Geometry check sheet. Reference: the model listing, model coordinates, mm. A direction names the side the tool comes from. Give positions to 0.01 mm unless a question says otherwise; leave off trailing zeros. Write each loop counter-clockwise with the first axis right and the second up, starting at its lowest first coordinate (ties: lowest second). Pieces come first, ordered by that corner, then holes. Notation, with made-up numbers: (82, 68.25) -> (114, 68.25) arc R20 cw to (114, 93.25) -> close; hole circle Ø5 at (38.25, 13). An arc over 180 degrees is marked (long way). One line per item, written item: value.
from build123d import *

# Parameters (mm, degrees)
F0_W      = 76.2
F0_H      = 38.1
F1_DEPTH  = 19.05
F3_DEPTH  = 3.048
F4_R      = 8.255
F5_DEPTH  = 4.572
F6_R      = 2.159
F7_DEPTH  = 12.7
F8_R      = 5.08
F9_DEPTH  = 12.7
F11_DEPTH = 3.048


with BuildPart() as f1:
    # F0 (on Top) → F1 (new body)
    with BuildSketch(Plane.XY):
        with Locations((38.1, 19.05)):
            Rectangle(F0_W, F0_H)
    extrude(amount=F1_DEPTH)

    # F2 (on face) → F3 (cut)
    with BuildSketch(Plane.XY.offset(19.05)):
        with BuildLine():
            ThreePointArc((7.0865621097, 27.8874175237), (11.4470908204, 28.4614920193), (13.4779330423, 32.3627036302))
            ThreePointArc((13.4779330423, 32.3627036302), (12.6166446532, 35.0943614084), (10.3443039749, 36.8379897367))
            ThreePointArc((10.3443039749, 36.8379897367), (4.2401469358, 33.9915745628), (7.0865621097, 27.8874175237))
        make_face()
        with BuildLine():
            ThreePointArc((10.3443039749, 36.8379897367), (12.6166446532, 35.0943614084), (13.4779330423, 32.3627036302))
            ThreePointArc((13.4779330423, 32.3627036302), (11.4470908204, 28.4614920193), (7.0865621097, 27.8874175237))
            Line((7.0865621097, 27.8874175237), (35.7283931912, 17.4626435552))
            ThreePointArc((35.7283931912, 17.4626435552), (32.5947641238, 21.9379296617), (35.7283931912, 26.4132157682))
            Line((35.7283931912, 26.4132157682), (37.3572641238, 27.0060763031))
            Line((37.3572641238, 27.0060763031), (10.3443039749, 36.8379897367))
        make_face()
        with BuildLine():
            Line((64.3702242728, 36.8379897367), (37.3572641238, 27.0060763031))
            Line((37.3572641238, 27.0060763031), (38.9861350564, 26.4132157682))
            ThreePointArc((38.9861350564, 26.4132157682), (41.2584757347, 24.6695874398), (42.1197641238, 21.9379296617))
            ThreePointArc((42.1197641238, 21.9379296617), (41.2584757347, 19.2062718836), (38.9861350564, 17.4626435552))
            Line((38.9861350564, 17.4626435552), (67.627966138, 27.8874175237))
            ThreePointArc((67.627966138, 27.8874175237), (61.5238090989, 30.7338326977), (64.3702242728, 36.8379897367))
        make_face()
        with BuildLine():
            Line((38.9861350564, 26.4132157682), (37.3572641238, 27.0060763031))
            Line((37.3572641238, 27.0060763031), (35.7283931912, 26.4132157682))
            ThreePointArc((35.7283931912, 26.4132157682), (37.3572641238, 26.7004296617), (38.9861350564, 26.4132157682))
        make_face()
        with BuildLine():
            ThreePointArc((35.7283931912, 26.4132157682), (32.5947641238, 21.9379296617), (35.7283931912, 17.4626435552))
            ThreePointArc((35.7283931912, 17.4626435552), (37.3572641238, 17.1754296617), (38.9861350564, 17.4626435552))
            ThreePointArc((38.9861350564, 17.4626435552), (41.2584757347, 19.2062718836), (42.1197641238, 21.9379296617))
            ThreePointArc((42.1197641238, 21.9379296617), (41.2584757347, 24.6695874398), (38.9861350564, 26.4132157682))
            ThreePointArc((38.9861350564, 26.4132157682), (37.3572641238, 26.7004296617), (35.7283931912, 26.4132157682))
        make_face()
        with BuildLine():
            ThreePointArc((70.7615952054, 32.3627036302), (68.7307529835, 36.2639152412), (64.3702242728, 36.8379897367))
            ThreePointArc((64.3702242728, 36.8379897367), (61.5238090989, 30.7338326977), (67.627966138, 27.8874175237))
            ThreePointArc((67.627966138, 27.8874175237), (69.9003068163, 29.6310458521), (70.7615952054, 32.3627036302))
        make_face()
    extrude(amount=-F3_DEPTH, mode=Mode.SUBTRACT)

    # F4 (on face) → F5 (cut)
    with BuildSketch(Plane.XY.offset(19.05)):
        with Locations((56.4142079383, 17.0484144696)):
            Circle(F4_R)
    extrude(amount=-F5_DEPTH, mode=Mode.SUBTRACT)

    # F6 (on face) → F7 (cut)
    with BuildSketch(Plane.XY.offset(14.478)):
        with Locations((56.4142079383, 17.0484144696)):
            Circle(F6_R)
    extrude(amount=-F7_DEPTH, mode=Mode.SUBTRACT)

    # F8 (on face) → F9 (cut)
    with BuildSketch(Plane.XY.offset(16.002)):
        with Locations((37.3572641238, 21.9379296617)):
            Circle(F8_R)
    extrude(amount=-F9_DEPTH, mode=Mode.SUBTRACT)

    # F10 (on face) → F11 (cut)
    with BuildSketch(Plane.XY.offset(19.05)):
        with BuildLine():
            ThreePointArc((7.0865621097, 27.8874175237), (4.8142214313, 29.6310458521), (3.9529330423, 32.3627036302))
            Line((3.9529330423, 32.3627036302), (3.9529330423, 0))
            Line((3.9529330423, 0), (70.7615952054, 0))
            Line((70.7615952054, 0), (70.7615952054, 32.3627036302))
            ThreePointArc((70.7615952054, 32.3627036302), (69.9003068163, 29.6310458521), (67.627966138, 27.8874175237))
            Line((67.627966138, 27.8874175237), (59.1989824769, 24.819518366))
            Line((59.1989824769, 24.819518366), (49.2857775794, 21.2114068571))
            Line((49.2857775794, 21.2114068571), (38.9861350564, 17.4626435552))
            ThreePointArc((38.9861350564, 17.4626435552), (37.3572641238, 17.1754296617), (35.7283931912, 17.4626435552))
            Line((35.7283931912, 17.4626435552), (7.0865621097, 27.8874175237))
        make_face()
    extrude(amount=-F11_DEPTH, mode=Mode.SUBTRACT)


solid = f1.part
1) Sectioned sample at C-C on z = 7. Record the cut outline in (x, y), plus the area to 3 significant figures.
Verdict:
outline: (0, 0) -> (76.2, 0) -> (76.2, 38.1) -> (0, 38.1) -> close; hole circle Ø10.16 at (37.36, 21.94); hole circle Ø4.32 at (56.41, 17.05)
area: 2,810 mm^2
2) Sectioned sample at B-B on y = 6.5. Record the cut outline in (x, z), plus the area to 3 significant figures.
Verdict:
outline: (0, 0) -> (76.2, 0) -> (76.2, 19.05) -> (70.76, 19.05) -> (70.76, 16) -> (3.95, 16) -> (3.95, 19.05) -> (0, 19.05) -> close
area: 1,250 mm^2
3) Mould release check, pull along Z, two halves, no side actions. Record for faces 4 (the flat face through (38, 19, 0)), 5 (the flat face through (24.04, 31.853, 17.547)), 6 (the flat face through (58, 15, 14.478)): released by +Z, released by -Z, zero draft, split by the parting line, or undercut.
Verdict:
face 4: released by -Z
face 5: zero draft
face 6: released by +Z
4) Sectioned sample at A-A on z = 18.25. Record the cut outline in (x, y) (1 decimal), plus the area to 3 significant figures.
Verdict:
outline: (0, 0) -> (4, 0) -> (4, 32.4) arc R4.8 cw to (10.3, 36.8) -> (37.4, 27) -> (64.4, 36.8) arc R4.8 cw to (70.8, 32.4) -> (70.8, 0) -> (76.2, 0) -> (76.2, 38.1) -> (0, 38.1) -> close
area: 714 mm^2
5) Depth check by flat-ended pin: pin 1 Ø5 at (x, y) = (53, 19) entering from +Z; pin 2 Ø5 at (x, y) = (37.5, 23) entering from +Z; pin 3 Ø3 at (x, y) = (32.5, 10.5) entering from +Z. Enter the tip coordinate at first touch or a pass-through.
Verdict:
pin 1: z = 14.48
pin 2: z = 3.3
pin 3: z = 16
6) Tool access check on faces 1 (the flat face through (38, 0, 9)), 2 (the flat face through (37, 15, 16.002)), 3 (the cylindrical face through (58.4, 16.2, 8.2)). Record the directions out of +Z, -Z, +X, -X, +Y, -Y that give a thin tool (end or side, any length) a straight path to the whole face; none if there is none.
Verdict:
face 1: +Z, -Z, +X, -X, -Y
face 2: +Z, -Y
face 3: +Z
7) Scan lines: probe 1 along Z at (x, y) = (53.5, 17); probe 2 along Y at (x, z) = (56, 6.5); probe 3 along Z at (x, y) = (62.5, 26.5). Record each from-to range of solid material in increasing order.
Verdict:
probe 1: 0 to 14.48
probe 2: 0 to 14.93, 19.17 to 38.1
probe 3: 0 to 16
8) Sectioned sample at D-D on x = 26.5. Record the cut outline in (y, z), plus the area to 3 significant figures.
Verdict:
outline: (0, 0) -> (38.1, 0) -> (38.1, 19.05) -> (30.96, 19.05) -> (30.96, 16) -> (0, 16) -> close
area: 631 mm^2
